from build123d import *

# Parameters (mm, degrees)
CROQUIS1_W                 = 75
CROQUIS1_H                 = 28
SALIENTE_EXTRUIR2_DEPTH    = 20
CROQUIS2_W                 = 75
CROQUIS2_H                 = 10
SALIENTE_EXTRUIR3_DEPTH    = 8.5
CROQUIS3_R                 = 2.4
CORTAR_EXTRUIR1_DEPTH      = 28
CROQUIS5_W                 = 3.5
CROQUIS5_H                 = 8
CORTAR_EXTRUIR2_DEPTH      = 12
REDONDEO1_R                = 18
CORTAR_EXTRUIR3_DEPTH      = 18.5
CORTAR_EXTRUIR3_DEPTH_BACK = 9.5
CROQUIS7_W                 = 50
CROQUIS7_H                 = 8.5
CROQUIS8_W                 = 50
CROQUIS8_H                 = 9
CORTAR_EXTRUIR4_DEPTH      = 20.5
REDONDEO2_R                = 10
REDONDEO5_R                = 10
CORTAR_EXTRUIR6_DEPTH      = 28.5
CROQUIS10_R                = 1.5
CORTAR_EXTRUIR7_DEPTH      = 85.977938313
REDONDEO6_R                = 10
REDONDEO7_R                = 3
REDONDEO8_R                = 5
CORTAR_EXTRUIR11_DEPTH     = 85.977938313
SALIENTE_EXTRUIR4_DEPTH    = 10
SALIENTE_EXTRUIR5_START    = -10
SALIENTE_EXTRUIR5_DEPTH    = 10
CORTAR_EXTRUIR12_START     = -0.5
CORTAR_EXTRUIR12_DEPTH     = 0.5
CROQUIS20_R                = 1.5
SALIENTE_EXTRUIR7_DEPTH    = 1
CORTAR_EXTRUIR13_DEPTH     = 85.977938313
CORTAR_EXTRUIR14_DEPTH     = 85.977938313
REDONDEO9_R                = 10


with BuildPart() as part:
    # Croquis1 → Saliente-Extruir2 (new body)
    with BuildSketch(Plane(origin=(0, 0, 0), x_dir=(1, 0, 0), z_dir=(0, 1, 0))):
        with Locations((37.5, 14)):
            Rectangle(CROQUIS1_W, CROQUIS1_H)
    extrude(amount=SALIENTE_EXTRUIR2_DEPTH)

    # Croquis2 → Saliente-Extruir3 (add)
    with BuildSketch(Plane(origin=(0, 20, 0), x_dir=(1, 0, 0), z_dir=(0, 1, 0))):
        with Locations((37.5, 5)):
            Rectangle(CROQUIS2_W, CROQUIS2_H)
        with Locations((37.5, 23)):
            Rectangle(CROQUIS2_W, CROQUIS2_H)
    extrude(amount=SALIENTE_EXTRUIR3_DEPTH)

    # Croquis3 → Cortar-Extruir1 (cut)
    with BuildSketch(Plane.XY):
        with Locations((63, 23.7)):
            Circle(CROQUIS3_R)
        with Locations((55, 23.7)):
            Circle(CROQUIS3_R)
    extrude(amount=-CORTAR_EXTRUIR1_DEPTH, mode=Mode.SUBTRACT)

    # Croquis5 → Cortar-Extruir2 (cut)
    with BuildSketch(Plane(origin=(0, 20, 0), x_dir=(1, 0, 0), z_dir=(0, 1, 0))):
        with Locations((73.25, 14)):
            Rectangle(CROQUIS5_W, CROQUIS5_H)
    extrude(amount=-CORTAR_EXTRUIR2_DEPTH, mode=Mode.SUBTRACT)

    # Redondeo1
    # the kernel refuses this fillet: 18 mm, written as the material it takes off along each edge
    with BuildSketch(Plane(origin=(71.5, 20, -10), x_dir=(0, -1, 0), z_dir=(0, 0, -1))) as redondeo1_piece_1:
        with BuildLine():
            CenterArc((18, 16.970562748), REDONDEO1_R, 180, 70.528779366)
            Line((0, 16.970562748), (0, 0))
            Line((0, 0), (12, 0))
        make_face()
    extrude(amount=8, mode=Mode.SUBTRACT)

    # Croquis7 → Cortar-Extruir3 (cut, two sides: drawn at the far end of the back side and taken through both)
    with BuildSketch(Plane.XY.offset(-18).offset(-CORTAR_EXTRUIR3_DEPTH_BACK)):
        with Locations((25, 24.25)):
            Rectangle(CROQUIS7_W, CROQUIS7_H)
    extrude(amount=CORTAR_EXTRUIR3_DEPTH + CORTAR_EXTRUIR3_DEPTH_BACK, mode=Mode.SUBTRACT)

    # Croquis8 → Cortar-Extruir4 (cut)
    with BuildSketch(Plane(origin=(0, 20, 0), x_dir=(1, 0, 0), z_dir=(0, 1, 0))):
        with Locations((25, 14.5)):
            Rectangle(CROQUIS8_W, CROQUIS8_H)
    extrude(amount=-CORTAR_EXTRUIR4_DEPTH, mode=Mode.SUBTRACT)

    # Redondeo2
    redondeo2_edges = [part.edges().sort_by_distance(p)[0] for p in [
        (0, 20, -5),
        (0, 20, -23.25),
    ]]
    fillet(redondeo2_edges, radius=REDONDEO2_R)

    # Redondeo5
    # the kernel refuses this fillet: 10 mm, written as the material it takes off along each edge
    with BuildSketch(Plane(origin=(0, 0, -35), x_dir=(1, 0, 0), z_dir=(0, 0, 1))) as redondeo5_piece_1:
        with BuildLine():
            CenterArc((REDONDEO5_R, REDONDEO5_R), REDONDEO5_R, 180, 90)
            Line((0, REDONDEO5_R), (0, 0))
            Line((0, 0), (REDONDEO5_R, 0))
        make_face()
    extrude(amount=60, mode=Mode.SUBTRACT)

    # Croquis9 → Cortar-Extruir6 (cut)
    with BuildSketch(Plane(origin=(0, 0, -28), x_dir=(-1, 0, 0), z_dir=(0, 0, -1))):
        with BuildLine():
            Line((-75, 28.5), (-59.5, 28.5))
            ThreePointArc((-59.5, 28.5), (-70.460155108, 23.960155108), (-75, 13))
            Line((-75, 13), (-75, 28.5))
        make_face()
    extrude(amount=-CORTAR_EXTRUIR6_DEPTH, mode=Mode.SUBTRACT)

    # Croquis10 → Cortar-Extruir7 (cut, through all)
    with BuildSketch(Plane(origin=(0, 0, -28), x_dir=(-1, 0, 0), z_dir=(0, 0, -1))):
        with Locations((-60.449874371, 9)):
            Circle(CROQUIS10_R)
        with Locations((-36.449874371, 9)):
            Circle(CROQUIS10_R)
        with Locations((-12.449874371, 9)):
            Circle(CROQUIS10_R)
    extrude(amount=-CORTAR_EXTRUIR7_DEPTH, mode=Mode.SUBTRACT)

    # Redondeo6
    redondeo6_edges = [part.edges().sort_by_distance(p)[0] for p in [
        (50, 0, -14.5),
    ]]
    fillet(redondeo6_edges, radius=REDONDEO6_R)

    # Redondeo7
    # the kernel refuses this fillet: 3 mm, written as the material it takes off along each edge
    with BuildSketch(Plane(origin=(50, 20, -18), x_dir=(0, -1, 0), z_dir=(0, 0, 1))) as redondeo7_piece_1:
        with BuildLine():
            CenterArc((REDONDEO7_R, REDONDEO7_R), REDONDEO7_R, 180, 90)
            Line((0, REDONDEO7_R), (0, 0))
            Line((0, 0), (REDONDEO7_R, 0))
        make_face()
    extrude(amount=8, mode=Mode.SUBTRACT)

    # Redondeo8
    redondeo8_edges = [part.edges().sort_by_distance(p)[0] for p in [
        (75, 0, -14),
    ]]
    fillet(redondeo8_edges, radius=REDONDEO8_R)

    # Croquis16 → Cortar-Extruir11 (cut, through all)
    with BuildSketch(Plane(origin=(0, 0, -28), x_dir=(-1, 0, 0), z_dir=(0, 0, -1))):
        with BuildLine():
            Line((-73.329316686, 20), (-69.329316686, 20))
            ThreePointArc((-69.329316686, 20), (-67.304546525, 25.119348054), (-62.716889054, 28.162507207))
            ThreePointArc((-62.716889054, 28.162507207), (-68.949863148, 25.286174608), (-73.329316686, 20))
        make_face()
    extrude(amount=-CORTAR_EXTRUIR11_DEPTH, mode=Mode.SUBTRACT)

    # Croquis17 → Saliente-Extruir4 (add)
    with BuildSketch(Plane(origin=(0, 0, -28), x_dir=(-1, 0, 0), z_dir=(0, 0, -1))):
        with BuildLine():
            Line((-73.329316686, 20), (-69.329316686, 20))
            ThreePointArc((-69.329316686, 20), (-67.839062436, 24.388682638), (-64.39628475, 27.491693244))
            ThreePointArc((-64.39628475, 27.491693244), (-69.382310449, 24.36530565), (-73.329316686, 20))
        make_face()
    extrude(amount=-SALIENTE_EXTRUIR4_DEPTH)

    # Croquis18 → Saliente-Extruir5 (add)
    with BuildSketch(Plane.XY.offset(SALIENTE_EXTRUIR5_START)):
        with BuildLine():
            ThreePointArc((64.39628475, 27.491693244), (67.839062436, 24.388682638), (69.329316686, 20))
            Line((69.329316686, 20), (73.329316686, 20))
            ThreePointArc((73.329316686, 20), (69.382310449, 24.36530565), (64.39628475, 27.491693244))
        make_face()
    extrude(amount=SALIENTE_EXTRUIR5_DEPTH)

    # Croquis19 → Cortar-Extruir12 (cut)
    with BuildSketch(Plane.XY.offset(-27.5).offset(CORTAR_EXTRUIR12_START)):
        with BuildLine():
            Line((50, 20), (50, 28.5))
            Line((50, 28.5), (0, 28.5))
            Line((0, 28.5), (0, 10))
            ThreePointArc((0, 10), (2.928932188, 17.071067812), (10, 20))
            Line((10, 20), (50, 20))
        make_face()
    extrude(amount=CORTAR_EXTRUIR12_DEPTH, mode=Mode.SUBTRACT)

    # Croquis20 → Saliente-Extruir7 (add)
    with BuildSketch(Plane.XY.offset(-19)):
        with BuildLine():
            Line((50, 20), (50, 10))
            ThreePointArc((50, 10), (52.928932188, 2.928932188), (60, 0))
            Line((60, 0), (10, 0))
            ThreePointArc((10, 0), (0, 10), (10, 20))
            Line((10, 20), (50, 20))
        make_face()
        with Locations(Location((12.449874371, 9, 0), (0, 0, 180))):
            Circle(CROQUIS20_R, mode=Mode.SUBTRACT)
        with Locations(Location((36.449874371, 9, 0), (0, 0, 180))):
            Circle(CROQUIS20_R, mode=Mode.SUBTRACT)
    extrude(amount=SALIENTE_EXTRUIR7_DEPTH)

    # Croquis21 → Cortar-Extruir13 (cut, through all)
    with BuildSketch(Plane.XY):
        with BuildLine():
            Line((10, 20), (36.449874371, 20))
            ThreePointArc((36.449874371, 20), (26.449874371, 10), (36.449874371, 0))
            Line((36.449874371, 0), (10, 0))
            ThreePointArc((10, 0), (0, 10), (10, 20))
        make_face()
    extrude(amount=-CORTAR_EXTRUIR13_DEPTH, mode=Mode.SUBTRACT)

    # Croquis22 → Cortar-Extruir14 (cut, through all)
    with BuildSketch(Plane.XY):
        with BuildLine():
            ThreePointArc((36.449874371, 0), (32.307738747, 10), (36.449874371, 20))
            ThreePointArc((36.449874371, 20), (26.449874371, 10), (36.449874371, 0))
        make_face()
    extrude(amount=-CORTAR_EXTRUIR14_DEPTH, mode=Mode.SUBTRACT)

    # Redondeo9
    # the kernel refuses this fillet: 10 mm, written as the material it takes off along each edge
    with BuildSketch(Plane(origin=(36.449874371, 20, 27.059805007), x_dir=(-0.3826834323650891, -0.9238795325112871, 0), z_dir=(0, 0, -1)), Plane(origin=(36.449874371, 20, 9.059805007), x_dir=(-0.3826834323650891, -0.9238795325112871, 0), z_dir=(0, 0, -1))) as redondeo9_piece_1:
        with BuildLine():
            CenterArc((6.997087679, -9.238795325), REDONDEO9_R, 67.5, 90)
            Line((-2.241707646, -5.411961001), (0, 0))
            ThreePointArc((0, 0), (5.411961001, 1.076505975), (10.823922003, 0))
        make_face()
    extrude(amount=64.119610015, mode=Mode.SUBTRACT)
    with BuildSketch(Plane(origin=(36.449874371, 0, 27.059805007), x_dir=(1, 0, 0), z_dir=(0, 0, -1)), Plane(origin=(36.449874371, 0, 9.059805007), x_dir=(1, 0, 0), z_dir=(0, 0, -1))) as redondeo9_piece_2:
        with BuildLine():
            CenterArc((5.857864376, -10), REDONDEO9_R, 90, 90)
            ThreePointArc((-4.142135624, -10), (-3.065629649, -4.588038999), (0, 0))
            Line((0, 0), (5.857864376, 0))
        make_face()
    extrude(amount=64.119610015, mode=Mode.SUBTRACT)


solid = part.part
Work out the finished part from the listing and answer in its coordinate system (mm). A direction names the side the tool comes from. Give positions to 0.01 mm unless a question says otherwise; leave off trailing zeros. Loops run counter-clockwise (first coordinate to the right, second up) from the corner with the lowest first, then second, coordinate; pieces in that order, holes last. Notation, with made-up numbers: M -0.5,-38.75 L 4.5,-38.75 A27 cw 4.5,-18.75 Z; hole C 51.25,60.5 d4. An arc over 180 degrees is marked long. Use CSV: the item, a comma, the result in double quotes.
1) Find section A-A on x = 43. Write down the section's boundary in (y, z).
Answer:
outline,"M 0,-28 L 20,-28 L 20,-18 L 0,-18 Z; M 0,-10 L 20,-10 L 20,0 L 0,0 Z"
2) Consider L1, parallel to Z at x = 58, y = 27.5; L2, parallel to Y at x = 55, z = -23.75; L3, parallel to Y at x = 53, z = -4.25. Determine where each line is inside the solid, lowest interval first.
Answer:
L1,"-28 to -18, -10 to 0"
L2,"0 to 21.3, 26.1 to 28.5"
L3,"0 to 22.37, 25.03 to 28.5"
3) Find section D-D on y = 25.5. Write down the section's boundary in (x, z), plus the area to 3 significant figures.
Answer:
outline,"M 50,-28 L 53.41,-28 L 53.41,-18 L 50,-18 Z; M 50,-10 L 53.41,-10 L 53.41,0 L 50,0 Z; M 56.59,-28 L 61.41,-28 L 61.41,-18 L 56.59,-18 Z; M 56.59,-10 L 61.41,-10 L 61.41,0 L 56.59,0 Z; M 64.59,-28 L 67.9,-28 L 67.9,-18 L 64.59,-18 Z; M 64.59,-10 L 67.9,-10 L 67.9,0 L 64.59,0 Z"
area,"231 mm^2"
4) Which of the six approach directions +Z, -Z, +X, -X, +Y, -Y give full straight-line access (tool end or side, diameter ignored) to faces 1 (the cylindrical face through (50.9, 19.14, -14.06)), 2 (the cylindrical face through (57.217, 22.781, -4.93)), 3 (the cylindrical face through (64.79, 16.79, -13.94)), 4 (the flat face through (46, 20, -23)), 5 (the cylindrical face through (74.565, 16.648, -23.07))?
Answer:
face 1,"-X, +Y"
face 2,"+Z, -Z"
face 3,"+X, +Y"
face 4,"+Z, -Z, -X, +Y"
face 5,"+Z, -Z, +X, +Y"
5) Find section C-C on y = 9. Write down the section's boundary in (x, z), plus the area to 3 significant figures.
Answer:
outline,"M 32.36,-28 L 34.95,-28 L 34.95,-18 L 32.36,-18 Z; M 32.36,-10 L 34.95,-10 L 34.95,0 L 32.36,0 Z; M 37.95,-28 L 58.95,-28 L 58.95,0 L 37.95,0 L 37.95,-10 L 50.05,-10 L 50.05,-18 L 37.95,-18 Z; M 61.95,-28 L 75,-28 L 75,-18 L 71.11,-18 L 71.11,-10 L 75,-10 L 75,0 L 61.95,0 Z"
area,"877 mm^2"
6) Find section B-B on z = -21.75. Write down the section's boundary in (x, y), plus the area to 3 significant figures.
Answer:
outline,"M 42.31,0 L 70,0 A5 ccw 75,5 L 75,13 A15.5 ccw 73.33,20 A21.42 ccw 64.4,27.49 A9.19 ccw 62.72,28.16 A15.5 ccw 59.5,28.5 L 50,28.5 L 50,20 L 42.31,20 A10 ccw Z; hole C 36.45,9 d3; hole C 55,23.7 d4.8; hole C 60.45,9 d3; hole C 63,23.7 d4.8"
area,"912 mm^2"
7) Determine the mould class of faces 6 (the cylindrical face through (37.64, 8.09, -5.07)), 7 (the cylindrical face through (32.31, 9.78, -22.93)), 8 (the cylindrical face through (61.09, 28.42, -5.07)) for opening direction X: released by +X, released by -X, zero draft, split by the parting line, or undercut.
Answer:
face 6,"undercut"
face 7,"released by -X"
face 8,"released by +X"
8) Given P1, Ø3, axis at x = 74, z = -13, coming from the +Y side; P2, Ø4, axis at y = 25.5, z = -5, coming from the -X side; P3, Ø14, axis at x = 43.5, y = 8, coming from the +Z side; P4, Ø5, axis at y = 18.5, z = -3, coming from the +X side, each flat-ended and moving along its own axis, determine where each tip first touches the part or whether it passes through.
Answer:
P1,"y = 8"
P2,"x = 50"
P3,"z = 0"
P4,"x = 74.71"
